from build123d import *

# Parameters (mm, degrees)
IZIM1_R                     = 27.5
IZIM1_R_2                   = 1.6
Y_KSEKLIK_EKSTR_ZYON1_DEPTH = 0.5


with BuildPart() as part:
    # Çizim1 → Yükseklik-Ekstrüzyon1 (new body)
    with BuildSketch(Plane.XY):
        Circle(IZIM1_R)
        with Locations((0, 24.7)):
            Circle(IZIM1_R_2, mode=Mode.SUBTRACT)
        with Locations((21.390827473, -12.35)):
            Circle(IZIM1_R_2, mode=Mode.SUBTRACT)
        with Locations((-21.390827473, -12.35)):
            Circle(IZIM1_R_2, mode=Mode.SUBTRACT)
        with BuildLine():
            Line((5.962564435, 13.127464544), (3.275, 14.679130594))
            ThreePointArc((3.275, 14.679130594), (2.542949192, 15.411181402), (2.275, 16.411181402))
            Line((2.275, 16.411181402), (2.275, 21.631617485))
            ThreePointArc((2.275, 21.631617485), (3.00525794, 23.176853746), (4.662755102, 23.593668957))
            ThreePointArc((4.662755102, 23.593668957), (12.025, 20.827910961), (18.101339134, 15.834898849))
            ThreePointArc((18.101339134, 15.834898849), (18.569115153, 14.191056594), (17.596030267, 12.786016536))
            Line((17.596030267, 12.786016536), (13.075, 10.175798494))
            ThreePointArc((13.075, 10.175798494), (12.075, 9.907849302), (11.075, 10.175798494))
            Line((11.075, 10.175798494), (8.387435565, 11.727464544))
            ThreePointArc((8.387435565, 11.727464544), (8.235671756, 11.747444629), (8.114230485, 11.654259464))
            Line((8.114230485, 11.654259464), (7.803105114, 11.115374514))
            ThreePointArc((7.803105114, 11.115374514), (7.780713917, 10.973636087), (7.859011515, 10.853383712))
            ThreePointArc((7.859011515, 10.853383712), (11.604740669, 6.699999553), (13.328811876, 1.379410738))
            ThreePointArc((13.328811876, 1.379410738), (13.393804684, 1.251476831), (13.527749366, 1.199998958))
            Line((13.527749366, 1.199998958), (14.15, 1.199998958))
            ThreePointArc((14.15, 1.199998958), (14.291421356, 1.258577601), (14.35, 1.399998958))
            Line((14.35, 1.399998958), (14.35, 4.5033321))
            ThreePointArc((14.35, 4.5033321), (14.617949192, 5.5033321), (15.35, 6.235382907))
            Line((15.35, 6.235382907), (19.871030267, 8.845600949))
            ThreePointArc((19.871030267, 8.845600949), (21.574373094, 8.985797151), (22.764094236, 7.758770109))
            ThreePointArc((22.764094236, 7.758770109), (24.05, 0), (22.764094236, -7.758770109))
            ThreePointArc((22.764094236, -7.758770109), (21.574373094, -8.985797151), (19.871030267, -8.845600949))
            Line((19.871030267, -8.845600949), (15.35, -6.235382907))
            ThreePointArc((15.35, -6.235382907), (14.617949192, -5.5033321), (14.35, -4.5033321))
            Line((14.35, -4.5033321), (14.35, -1.400001042))
            ThreePointArc((14.35, -1.400001042), (14.291421356, -1.258579686), (14.15, -1.200001042))
            Line((14.15, -1.200001042), (13.527749151, -1.200001042))
            ThreePointArc((13.527749151, -1.200001042), (13.393804479, -1.251478906), (13.328811663, -1.379412792))
            ThreePointArc((13.328811663, -1.379412792), (11.604739636, -6.700001341), (7.859009843, -10.853384923))
            ThreePointArc((7.859009843, -10.853384923), (7.780712223, -10.973637301), (7.803103416, -11.115375743))
            Line((7.803103416, -11.115375743), (8.114228679, -11.654260506))
            ThreePointArc((8.114228679, -11.654260506), (8.235669951, -11.747445671), (8.38743376, -11.727465587))
            Line((8.38743376, -11.727465587), (11.075, -10.175798494))
            ThreePointArc((11.075, -10.175798494), (12.075, -9.907849302), (13.075, -10.175798494))
            Line((13.075, -10.175798494), (17.596030267, -12.786016536))
            ThreePointArc((17.596030267, -12.786016536), (18.569115153, -14.191056594), (18.101339134, -15.834898849))
            ThreePointArc((18.101339134, -15.834898849), (12.025, -20.827910961), (4.662755102, -23.593668957))
            ThreePointArc((4.662755102, -23.593668957), (3.00525794, -23.176853746), (2.275, -21.631617485))
            Line((2.275, -21.631617485), (2.275, -16.411181402))
            ThreePointArc((2.275, -16.411181402), (2.542949192, -15.411181402), (3.275, -14.679130594))
            Line((3.275, -14.679130594), (5.962562629, -13.127465587))
            ThreePointArc((5.962562629, -13.127465587), (6.055747795, -13.006024315), (6.03576771, -12.854260506))
            Line((6.03576771, -12.854260506), (5.724642232, -12.315375369))
            ThreePointArc((5.724642232, -12.315375369), (5.613088766, -12.225114815), (5.469798369, -12.23279632))
            ThreePointArc((5.469798369, -12.23279632), (-2.065e-06, -13.4), (-5.469802139, -12.232794634))
            ThreePointArc((-5.469802139, -12.232794634), (-5.613092563, -12.225113095), (-5.724646058, -12.315373658))
            Line((-5.724646058, -12.315373658), (-6.035771321, -12.854258421))
            ThreePointArc((-6.035771321, -12.854258421), (-6.055751405, -13.00602223), (-5.96256624, -13.127463502))
            Line((-5.96256624, -13.127463502), (-3.275, -14.679130594))
            ThreePointArc((-3.275, -14.679130594), (-2.542949192, -15.411181402), (-2.275, -16.411181402))
            Line((-2.275, -16.411181402), (-2.275, -21.631617485))
            ThreePointArc((-2.275, -21.631617485), (-3.00525794, -23.176853746), (-4.662755102, -23.593668957))
            ThreePointArc((-4.662755102, -23.593668957), (-12.025, -20.827910961), (-18.101339134, -15.834898849))
            ThreePointArc((-18.101339134, -15.834898849), (-18.569115153, -14.191056594), (-17.596030267, -12.786016536))
            Line((-17.596030267, -12.786016536), (-13.075, -10.175798494))
            ThreePointArc((-13.075, -10.175798494), (-12.075, -9.907849302), (-11.075, -10.175798494))
            Line((-11.075, -10.175798494), (-8.387437371, -11.727463502))
            ThreePointArc((-8.387437371, -11.727463502), (-8.235673562, -11.747443587), (-8.11423229, -11.654258421))
            Line((-8.11423229, -11.654258421), (-7.803106811, -11.115373285))
            ThreePointArc((-7.803106811, -11.115373285), (-7.780715611, -10.973634873), (-7.859013188, -10.853382501))
            ThreePointArc((-7.859013188, -10.853382501), (-11.604741185, -6.699998659), (-13.328811876, -1.379410738))
            ThreePointArc((-13.328811876, -1.379410738), (-13.393804684, -1.251476831), (-13.527749366, -1.199998958))
            Line((-13.527749366, -1.199998958), (-14.15, -1.199998958))
            ThreePointArc((-14.15, -1.199998958), (-14.291421356, -1.258577601), (-14.35, -1.399998958))
            Line((-14.35, -1.399998958), (-14.35, -4.5033321))
            ThreePointArc((-14.35, -4.5033321), (-14.617949192, -5.5033321), (-15.35, -6.235382907))
            Line((-15.35, -6.235382907), (-19.871030267, -8.845600949))
            ThreePointArc((-19.871030267, -8.845600949), (-21.574373094, -8.985797151), (-22.764094236, -7.758770109))
            ThreePointArc((-22.764094236, -7.758770109), (-24.05, 0), (-22.764094236, 7.758770109))
            ThreePointArc((-22.764094236, 7.758770109), (-21.574373094, 8.985797151), (-19.871030267, 8.845600949))
            Line((-19.871030267, 8.845600949), (-15.35, 6.235382907))
            ThreePointArc((-15.35, 6.235382907), (-14.617949192, 5.5033321), (-14.35, 4.5033321))
            Line((-14.35, 4.5033321), (-14.35, 1.400001042))
            ThreePointArc((-14.35, 1.400001042), (-14.291421356, 1.258579686), (-14.15, 1.200001042))
            Line((-14.15, 1.200001042), (-13.527749151, 1.200001042))
            ThreePointArc((-13.527749151, 1.200001042), (-13.393804479, 1.251478906), (-13.328811663, 1.379412792))
            ThreePointArc((-13.328811663, 1.379412792), (-11.604740153, 6.700000447), (-7.859011515, 10.853383712))
            ThreePointArc((-7.859011515, 10.853383712), (-7.780713917, 10.973636087), (-7.803105114, 11.115374514))
            Line((-7.803105114, 11.115374514), (-8.114230485, 11.654259464))
            ThreePointArc((-8.114230485, 11.654259464), (-8.235671756, 11.747444629), (-8.387435565, 11.727464544))
            Line((-8.387435565, 11.727464544), (-11.075, 10.175798494))
            ThreePointArc((-11.075, 10.175798494), (-12.075, 9.907849302), (-13.075, 10.175798494))
            Line((-13.075, 10.175798494), (-17.596030267, 12.786016536))
            ThreePointArc((-17.596030267, 12.786016536), (-18.569115153, 14.191056594), (-18.101339134, 15.834898849))
            ThreePointArc((-18.101339134, 15.834898849), (-15.719264288, 18.201846891), (-13.030721544, 20.213925795))
            ThreePointArc((-13.030721544, 20.213925795), (-12.948542196, 20.32125171), (-12.953404277, 20.456339302))
            ThreePointArc((-12.953404277, 20.456339302), (-12.525, 21.693936365), (-11.239007365, 21.44614682))
            ThreePointArc((-11.239007365, 21.44614682), (-11.12444912, 21.374392338), (-10.990412477, 21.391898784))
            ThreePointArc((-10.990412477, 21.391898784), (-7.903629659, 22.714205648), (-4.662755102, 23.593668957))
            ThreePointArc((-4.662755102, 23.593668957), (-3.00525794, 23.176853746), (-2.275, 21.631617485))
            Line((-2.275, 21.631617485), (-2.275, 16.411181402))
            ThreePointArc((-2.275, 16.411181402), (-2.542949192, 15.411181402), (-3.275, 14.679130594))
            Line((-3.275, 14.679130594), (-5.962564435, 13.127464544))
            ThreePointArc((-5.962564435, 13.127464544), (-6.0557496, 13.006023273), (-6.035769515, 12.854259464))
            Line((-6.035769515, 12.854259464), (-5.724644145, 12.315374514))
            ThreePointArc((-5.724644145, 12.315374514), (-5.613090664, 12.225113955), (-5.469800254, 12.232795477))
            ThreePointArc((-5.469800254, 12.232795477), (0, 13.4), (5.469800254, 12.232795477))
            ThreePointArc((5.469800254, 12.232795477), (5.613090664, 12.225113955), (5.724644145, 12.315374514))
            Line((5.724644145, 12.315374514), (6.035769515, 12.854259464))
            ThreePointArc((6.035769515, 12.854259464), (6.0557496, 13.006023273), (5.962564435, 13.127464544))
        make_face(mode=Mode.SUBTRACT)
    extrude(amount=Y_KSEKLIK_EKSTR_ZYON1_DEPTH)


solid = part.part
Could you check a few things on this model? Use its own coordinates, in mm. Round coordinates to 2 decimals unless told otherwise and drop trailing zeros. Write each loop counter-clockwise with the first axis right and the second up, starting at its lowest first coordinate (ties: lowest second). Pieces come first, ordered by that corner, then holes. Notation, with made-up numbers: (-25.5, 5.5) - (17.5, 5.5) arc R33 cw to (17.5, 38.5) - close; hole circle Ø10 at (65, 10.5). An arc over 180 degrees is marked (long way). Use a Markdown table: item, result.
Q1. I want a section at A-A (x = 0). List the corners of the cut face in (y, z) for me.
Output values:
| item | result |
|---|---|
| outline | (-27.5, 0) - (-13.4, 0) - (-13.4, 0.5) - (-27.5, 0.5) - close; (13.4, 0) - (23.1, 0) - (23.1, 0.5) - (13.4, 0.5) - close; (26.3, 0) - (27.5, 0) - (27.5, 0.5) - (26.3, 0.5) - close |
Q2. I want a section at B-B (y = 0). List the corners of the cut face in (x, z) for me.
Output values:
| item | result |
|---|---|
| outline | (-27.5, 0) - (-24.05, 0) - (-24.05, 0.5) - (-27.5, 0.5) - close; (24.05, 0) - (27.5, 0) - (27.5, 0.5) - (24.05, 0.5) - close |
Q3. I want a section at D-D (y = 24.7). List the corners of the cut face in (x, z) for me.
Output values:
| item | result |
|---|---|
| outline | (-12.09, 0) - (-1.6, 0) - (-1.6, 0.5) - (-12.09, 0.5) - close; (1.6, 0) - (12.09, 0) - (12.09, 0.5) - (1.6, 0.5) - close |
Q4. Thinking about a two-plate mould opening in Y: for faces 1 (the flat face through (10, -10, 0)), 2 (the cylindrical face through (-5.961, -26.846, 0.246)), 3 (the cylindrical face through (24.05, 0.11, 0.25)), which applies, released by +Y, released by -Y, zero draft, split by the parting line, or undercut?
Output values:
| item | result |
|---|---|
| face 1 | zero draft |
| face 2 | split by the parting line |
| face 3 | undercut |
Q5. I want a section at C-C (y = 18.5). List the corners of the cut face in (x, z) for me (3 decimals).
Output values:
| item | result |
|---|---|
| outline | (-20.347, 0) - (-15.367, 0) - (-15.367, 0.5) - (-20.347, 0.5) - close; (-2.275, 0) - (2.275, 0) - (2.275, 0.5) - (-2.275, 0.5) - close; (15.367, 0) - (20.347, 0) - (20.347, 0.5) - (15.367, 0.5) - close |
Q6. Please list where these lines run through material, in increasing order: L1, parallel to Y at x = 0, z = 0.35; L2, parallel to X at y = 18, z = 0.25 (3 decimals); L3, parallel to X at y = -3, z = 0.1.
Output values:
| item | result |
|---|---|
| L1 | -27.5 to -13.4, 13.4 to 23.1, 26.3 to 27.5 |
| L2 | -20.791 to -15.95, -2.275 to 2.275, 15.95 to 20.791 |
| L3 | -27.34 to -23.86, -14.35 to -13.06, 13.06 to 14.35, 23.86 to 27.34 |
